from build123d import *

# Parameters (mm, degrees)
F0_W     = 146.05
F0_H     = 90
F0_R     = 4.5
F0_R_2   = 2.25
F1_DEPTH = 6
F2_DEPTH = 3.5
F3_W     = 90
F3_H     = 14
F3_R     = 1.25
F4_DEPTH = 5
F5_W     = 90
F5_H     = 8
F5_R     = 1.25
F6_DEPTH = 5


with BuildPart() as f1:
    # F0 (on Top) → F1 (new body)
    with BuildSketch(Plane.XY):
        Rectangle(F0_W, F0_H)
        with Locations((-47.625, -38.1)):
            Circle(F0_R, mode=Mode.SUBTRACT)
        with Locations((47.625, -38.1)):
            Circle(F0_R, mode=Mode.SUBTRACT)
        with Locations((-47.625, 38.1)):
            Circle(F0_R, mode=Mode.SUBTRACT)
        with Locations((47.625, 38.1)):
            Circle(F0_R, mode=Mode.SUBTRACT)
        with Locations((-47.625, 38.1)):
            Circle(F0_R)
        with Locations((-47.625, 38.1)):
            Circle(F0_R_2, mode=Mode.SUBTRACT)
        with Locations((-47.625, -38.1)):
            Circle(F0_R)
        with Locations((-47.625, -38.1)):
            Circle(F0_R_2, mode=Mode.SUBTRACT)
        with Locations((47.625, -38.1)):
            Circle(F0_R)
        with Locations((47.625, -38.1)):
            Circle(F0_R_2, mode=Mode.SUBTRACT)
        with Locations((47.625, 38.1)):
            Circle(F0_R)
        with Locations((47.625, 38.1)):
            Circle(F0_R_2, mode=Mode.SUBTRACT)
    extrude(amount=F1_DEPTH)

    # F0 (on Top) → F2 (cut)
    with BuildSketch(Plane.XY):
        with Locations((-47.625, 38.1)):
            Circle(F0_R)
        with Locations((-47.625, 38.1)):
            Circle(F0_R_2, mode=Mode.SUBTRACT)
        with Locations((-47.625, -38.1)):
            Circle(F0_R)
        with Locations((-47.625, -38.1)):
            Circle(F0_R_2, mode=Mode.SUBTRACT)
        with Locations((47.625, -38.1)):
            Circle(F0_R)
        with Locations((47.625, -38.1)):
            Circle(F0_R_2, mode=Mode.SUBTRACT)
        with Locations((47.625, 38.1)):
            Circle(F0_R)
        with Locations((47.625, 38.1)):
            Circle(F0_R_2, mode=Mode.SUBTRACT)
    extrude(amount=F2_DEPTH, mode=Mode.SUBTRACT)

    # F3 (on face) → F4 (join)
    with BuildSketch(Plane.YZ.offset(73.025)):
        with Locations((0, 7)):
            Rectangle(F3_W, F3_H)
        with Locations((-39.625, 10)):
            Circle(F3_R, mode=Mode.SUBTRACT)
        with Locations((39.625, 10)):
            Circle(F3_R, mode=Mode.SUBTRACT)
    extrude(amount=-F4_DEPTH)

    # F5 (on face) → F6 (join)
    with BuildSketch(Plane(origin=(-73.025, 0, 0), x_dir=(0, -1, 0), z_dir=(-1, 0, 0))):
        with Locations((0, 10)):
            Rectangle(F5_W, F5_H)
        with Locations((-39.625, 10)):
            Circle(F5_R, mode=Mode.SUBTRACT)
        with Locations((39.625, 10)):
            Circle(F5_R, mode=Mode.SUBTRACT)
    extrude(amount=-F6_DEPTH)


solid = f1.part
The model under review builds one solid part; all positions refer to its coordinate system, in mm. A direction names the side the tool comes from. Give positions to 0.01 mm unless a question says otherwise; leave off trailing zeros. Loops run counter-clockwise (first coordinate to the right, second up) from the corner with the lowest first, then second, coordinate; pieces in that order, holes last. Notation, with made-up numbers: (-16.75, -25.5) -> (0.25, -25.5) arc R29 ccw to (0.25, -5.5) -> close; hole circle Ø5 at (21, 8.25). An arc over 180 degrees is marked (long way). Put each result on its own line as item: value. Start each with the question number.
1. We need section B-B on y = 1.5. State the section outline as (x, z) points (3 decimals), then the cut area to 3 significant figures.
2. Wall thickness on probe 1 along Y at (x, z) = (-48.5, 3); probe 2 along X at (y, z) = (41, 8) (3 decimals); probe 3 along Z at (x, y) = (51, -21): over which ranges is each line inside the solid? List them lowest first.
3. Mouldability with a two-part tool opening along X and no side actions: class faces 1 (the face through (-1, 1, 0)), 2 (the face through (49.701, 34.108, 1.726)), 3 (the face through (-45.549, 34.108, 1.726)), 4 (the face through (-73.025, 1, 7)) as released by +X, released by -X, zero draft, split by the parting line, or undercut.
4. We need section A-A on z = 2. State the section outline as (x, y) points (3 decimals), then the cut area to 3 significant figures.
5. Clearance check with flat-ended pins moving along their axes: P1, Ø11.5, axis at x = -47.625, y = -38.1, coming from the +Z side; P2, Ø2.5, axis at x = -49, y = -36.5, coming from the -Z side; P3, Ø4, axis at y = 39.625, z = 10, coming from the +X side (3 decimals); P4, Ø2, axis at y = 39.625, z = 10, coming from the +X side. State where each tip first meets the part, or that it passes through.
6. For faces 5 (the face through (-49.3, 39.6, 4.7)), 6 (the face through (-45.549, -42.092, 1.726)), 7 (the face through (-68.025, 1, 10)), list the 3-axis set-ups (+Z, -Z, +X, -X, +Y, -Y) from which the entire face can be reached by the end or side of a thin tool; tool diameter is ignored.
7. We need section C-C on x = -26. State the section outline as (y, z) points.
Determined:
1. outline: (-73.025, 0) -> (73.025, 0) -> (73.025, 14) -> (68.025, 14) -> (68.025, 6) -> (-68.025, 6) -> (-68.025, 14) -> (-73.025, 14) -> close
1. area: 956 mm^2
2. probe 1: -45 to -42.51, -33.69 to 33.69, 42.51 to 45
2. probe 2: -73.025 to -68.025, 68.025 to 73.025
2. probe 3: 0 to 6
3. face 1: zero draft
3. face 2: undercut
3. face 3: undercut
3. face 4: released by -X
4. outline: (-73.025, -45) -> (73.025, -45) -> (73.025, 45) -> (-73.025, 45) -> close; hole circle Ø9 at (-47.625, -38.1); hole circle Ø9 at (-47.625, 38.1); hole circle Ø9 at (47.625, -38.1); hole circle Ø9 at (47.625, 38.1)
4. area: 12,900 mm^2
5. P1: z = 6
5. P2: z = 3.5
5. P3: x = 73.025
5. P4: through
6. face 5: +Z, -Z
6. face 6: -Z
6. face 7: +Z, +Y, -Y
7. outline: (-45, 0) -> (45, 0) -> (45, 6) -> (-45, 6) -> close
